from build123d import *

# Parameters (mm, degrees)
BOSS_EXTRU_1_DEPTH      = 20
ENL_V_MAT_EXTRU_1_DEPTH = 8
ESQUISSE3_R             = 15
ESQUISSE3_R_2           = 10
ENL_V_MAT_EXTRU_2_DEPTH = 115.149577324


with BuildPart() as part:
    # Esquisse1 → Boss.-Extru.1 (new, symmetric)
    with BuildSketch(Plane(origin=(0, 0, 0), x_dir=(1, 0, 0), z_dir=(0, 1, 0))):
        with BuildLine():
            Line((0, 0), (50, 0))
            Line((50, 0), (79.69848481, 29.69848481))
            ThreePointArc((79.69848481, 29.69848481), (82.04163056, 35.355339059), (79.69848481, 41.012193309))
            Line((79.69848481, 41.012193309), (46.246943589, 74.463734529))
            ThreePointArc((46.246943589, 74.463734529), (38.809068701, 76.606108799), (33.038444811, 71.447460693))
            ThreePointArc((33.038444811, 71.447460693), (20.256617737, 54.457585283), (0, 48))
            ThreePointArc((0, 48), (-14, 34), (0, 20))
            Line((0, 20), (0, 0))
        make_face()
    extrude(amount=BOSS_EXTRU_1_DEPTH, both=True)

    # Esquisse2 → Enlèv. mat.-Extru.1 (cut)
    with BuildSketch(Plane(origin=(0, 20, 0), x_dir=(1, 0, 0), z_dir=(0, 1, 0))):
        with BuildLine():
            Line((20, 40.573593129), (20, 10))
            ThreePointArc((20, 10), (18.535533906, 6.464466094), (15, 5))
            Line((15, 5), (10, 5))
            ThreePointArc((10, 5), (6.464466094, 6.464466094), (5, 10))
            Line((5, 10), (5, 20))
            ThreePointArc((5, 20), (3.535533906, 23.535533906), (0, 25))
            ThreePointArc((0, 25), (-9, 34), (0, 43))
            ThreePointArc((0, 43), (6.764079149, 43.576057614), (13.333333333, 45.287638337))
            ThreePointArc((13.333333333, 45.287638337), (17.886751346, 44.656076033), (20, 40.573593129))
        make_face()
    extrude(amount=-ENL_V_MAT_EXTRU_1_DEPTH, mode=Mode.SUBTRACT)

    # Esquisse3 → Enlèv. mat.-Extru.2 (cut, through all)
    with BuildSketch(Plane.XY):
        with Locations(Location((50, 0, 0), (0, 0, 270))):
            Circle(ESQUISSE3_R)
        with Locations((-14, 0)):
            Circle(ESQUISSE3_R_2)
    extrude(amount=-ENL_V_MAT_EXTRU_2_DEPTH, mode=Mode.SUBTRACT)


solid = part.part
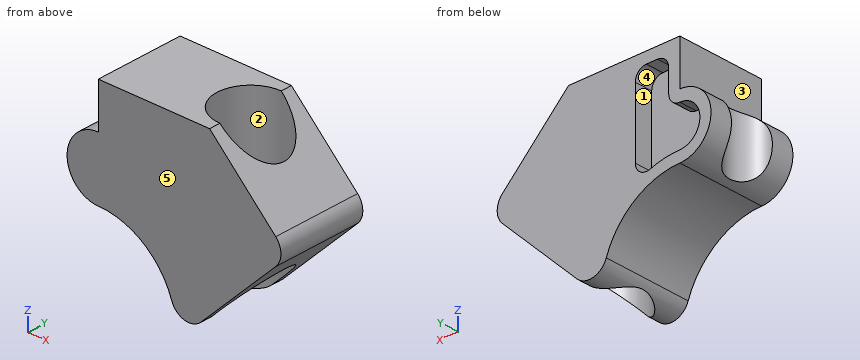
Model file for the job. Use its own axes, mm. Face numbers are marked on the shaded views. A direction names the side the tool comes from. Coordinates: 2 decimals unless noted, no trailing zeros. Write each loop counter-clockwise with the first axis right and the second up, starting at its lowest first coordinate (ties: lowest second). Pieces come first, ordered by that corner, then holes. Notation, with made-up numbers: (-19.5, 52) -> (-8.5, 52) arc R31 cw to (-8.5, 85) -> close; hole circle Ø10 at (-17.75, 74). An arc over 180 degrees is marked (long way). One line per item, written item: value. Start each with the question number.
1) Pull direction X, two halves, no side cores. Call the marked faces 3, 4 and 5: +X half, -X half, draft (parallel to the pull), parting line (faces both ways), or undercut.
2) Slice it at B-B on y = 0. Write the cut outline in (x, z), then the cut area to 3 significant figures.
3) Which spindle directions (+Z, -Z, +X, -X, +Y, -Y) get a long thin tool onto all of the face, cutting with end or side? Do the marked faces 1 and 2. Say none if no direction does.
4) Slice it at C-C on z = -34. Write the cut outline in (x, y).
5) Slice it at A-A on x = 62. Write the cut outline in (y, z), then the cut area to 3 significant figures.
6) Slice it at D-D on x = -2. Write the cut outline in (y, z), then the cut area to 3 significant figures.
7) Probe probe 1 along Y at (x, z) = (50, -18); probe 2 along X at (y, z) = (13.5, -17); probe 3 along X at (y, z) = (-6, -53.5). List the from-to ranges inside material, lowest first.
8) Flat gauge pins, fed straight in: pin 1 Ø1 at (x, y) = (2, -16) entering from -Z; pin 2 Ø3 at (x, y) = (72, 6.5) entering from -Z; pin 3 Ø1.5 at (x, y) = (13.5, 15.5) entering from -Z; pin 4 Ø24 at (x, y) = (50, 0) entering from -Z. Where does each tip first touch, or does it go through?
Answers follow:
1. face 3: -X half
1. face 4: undercut
1. face 5: draft
2. outline: (-4, -47.42) arc R14 ccw to (0, -48) arc R35 cw to (33.04, -71.45) arc R8 ccw to (35, -74.53) -> (35, 0) -> (0, 0) -> (0, -20) arc R14 ccw to (-4, -20.58) -> close; (65, -55.71) -> (79.7, -41.01) arc R8 ccw to (79.7, -29.7) -> (65, -15) -> close
2. area: 2,450 mm2
3. face 1: +Y
3. face 2: +Z, -Z
4. outline: (-14, -20) -> (81.93, -20) -> (81.93, 20) -> (20, 20) -> (20, 12) -> (-9, 12) -> (-9, 20) -> (-14, 20) -> (-14, 10) arc R10 cw to (-14, -10) -> close; hole circle Ø30 at (50, 0)
5. outline: (-20, -58.71) -> (-9, -58.71) -> (-9, -12) -> (-20, -12) -> close; (9, -58.71) -> (20, -58.71) -> (20, -12) -> (9, -12) -> close
5. area: 1,030 mm2
6. outline: (-20, -47.86) -> (20, -47.86) -> (20, -42.77) -> (12, -42.77) -> (12, -25.23) -> (20, -25.23) -> (20, -20.14) -> (-20, -20.14) -> close
6. area: 968 mm2
7. probe 1: -20 to -15, 15 to 20
7. probe 2: 0 to 5, 20 to 43.46, 56.54 to 67
7. probe 3: 18.83 to 36.25, 63.75 to 67.21
8. pin 1: z = -48.09
8. pin 2: z = -50.21
8. pin 3: z = -51.03
8. pin 4: through
